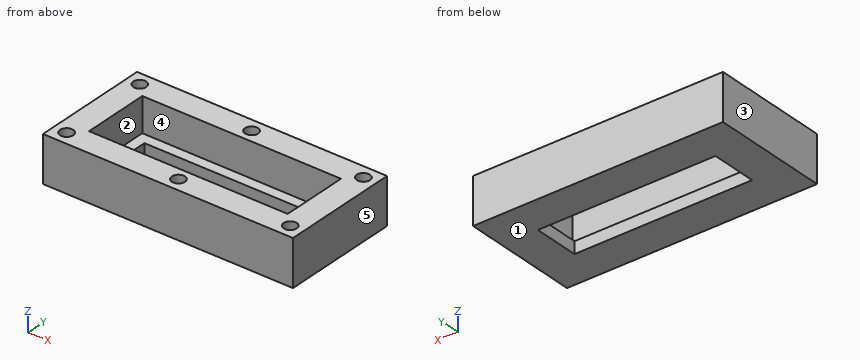
```python
from build123d import *

# Parameters (mm, degrees)
F0_W     = 241.3
F0_H     = 114.3
F1_DEPTH = 44.45
F2_W     = 191.77
F2_H     = 64.77
F3_DEPTH = 33.02
F4_W     = 171.45
F4_H     = 44.45
F5_DEPTH = 25.4
F6_R     = 6.35
F7_DEPTH = 25.4


with BuildPart() as f1:
    # F0 (on Top) → F1 (new body)
    with BuildSketch(Plane.XY):
        Rectangle(F0_W, F0_H)
    extrude(amount=F1_DEPTH)

    # F2 (on face) → F3 (cut)
    with BuildSketch(Plane.XY.offset(44.45)):
        Rectangle(F2_W, F2_H)
    extrude(amount=-F3_DEPTH, mode=Mode.SUBTRACT)

    # F4 (on face) → F5 (cut)
    with BuildSketch(Plane(origin=(0, 0, 0), x_dir=(1, 0, 0), z_dir=(0, 0, -1))):
        Rectangle(F4_W, F4_H)
    extrude(amount=-F5_DEPTH, mode=Mode.SUBTRACT)

    # F6 (on face) → F7 (cut)
    with BuildSketch(Plane.XY.offset(44.45)):
        with Locations((-107.95, 44.45)):
            Circle(F6_R)
        with Locations((0, 44.45)):
            Circle(F6_R)
        with Locations((107.95, 44.45)):
            Circle(F6_R)
        with Locations((107.95, -44.45)):
            Circle(F6_R)
        with Locations((0, -44.45)):
            Circle(F6_R)
        with Locations((-107.95, -44.45)):
            Circle(F6_R)
    extrude(amount=-F7_DEPTH, mode=Mode.SUBTRACT)


solid = f1.part
```
Could you check a few things on this model? Use its own coordinates, in mm. Face numbers are marked on the shaded views. A direction names the side the tool comes from. Coordinates: 2 decimals unless noted, no trailing zeros. Write each loop counter-clockwise with the first axis right and the second up, starting at its lowest first coordinate (ties: lowest second). Pieces come first, ordered by that corner, then holes. Notation, with made-up numbers: M -19.5,22.25 L 39.5,22.25 A21 cw 39.5,53.25 Z; hole C 54,24.25 d4. An arc over 180 degrees is marked long. Answer as CSV lines item,"result". Start each with the question number.
1) We'd pull the mould along X, two halves only. Please class the marked faces 1, 2 and 3: +X half, -X half, draft (parallel to the pull), parting line (faces both ways), or undercut.
2) I want a section at B-B, the plane z = 29. Please give me the cut outline in (x, y) (3 decimals).
3) Please list where these lines run through material, in increasing order: line 1 (Y direction, x = 0, z = 25.25) (3 decimals); line 2 (X direction, y = 44, z = 28); line 3 (Y direction, x = -86, z = 15) (3 decimals). Write a range as from..to.
4) I want a section at C-C, the plane x = -29. Please give me the cut outline in (y, z) (3 decimals), and give its area (3 significant figures).
5) For the marked faces 4 and 5, which set-ups out of +Z, -Z, +X, -X, +Y, -Y let a thin tool reach every point of the face, with its end or its side?
6) For P1, Ø12, axis at x = 40.5, y = -21, coming from the +Z side; P2, Ø6.5, axis at x = 107.5, y = 44, coming from the +Z side, each with a flat end and sliding along its axis, tell me the tip position at first contact or that it passes through.
7) I want a section at D-D, the plane x = -107.95. Please give me the cut outline in (y, z).
8) I want a section at A-A, the plane y = -4. Please give me the cut outline in (x, z) (3 decimals).
Data:
1,face 1,"draft"
1,face 2,"undercut"
1,face 3,"-X half"
2,outline,"M -120.65,-57.15 L 120.65,-57.15 L 120.65,57.15 L -120.65,57.15 Z; hole C -107.95,-44.45 d12.7; hole C -107.95,44.45 d12.7; hole M -95.885,-32.385 L 95.885,-32.385 L 95.885,32.385 L -95.885,32.385 Z; hole C 0,-44.45 d12.7; hole C 0,44.45 d12.7; hole C 107.95,-44.45 d12.7; hole C 107.95,44.45 d12.7"
3,line 1,"y = -57.15..-50.8, -38.1..-32.385, 32.385..38.1, 50.8..57.15"
3,line 2,"x = -120.65..-114.28, -101.62..-6.33, 6.33..101.62, 114.28..120.65"
3,line 3,"y = -57.15..-32.385, 32.385..57.15"
4,outline,"M -57.15,0 L -22.225,0 L -22.225,11.43 L -32.385,11.43 L -32.385,44.45 L -57.15,44.45 Z; M 22.225,0 L 57.15,0 L 57.15,44.45 L 32.385,44.45 L 32.385,11.43 L 22.225,11.43 Z"
4,area,"2,430 mm^2"
5,face 4,"+Z"
5,face 5,"+Z, -Z, +X, +Y, -Y"
6,P1,"stops at z = 11.43"
6,P2,"stops at z = 19.05"
7,outline,"M -57.15,0 L 57.15,0 L 57.15,44.45 L 50.8,44.45 L 50.8,19.05 L 38.1,19.05 L 38.1,44.45 L -38.1,44.45 L -38.1,19.05 L -50.8,19.05 L -50.8,44.45 L -57.15,44.45 Z"
8,outline,"M -120.65,0 L -85.725,0 L -85.725,11.43 L -95.885,11.43 L -95.885,44.45 L -120.65,44.45 Z; M 85.725,0 L 120.65,0 L 120.65,44.45 L 95.885,44.45 L 95.885,11.43 L 85.725,11.43 Z"
